from build123d import *

# Parameters (mm, degrees)
SKETCH1_R           = 4
BOSS_EXTRUDE1_DEPTH = 203.2
SKETCH2_R           = 1.864950538
CUT_EXTRUDE1_DEPTH  = 12.7
CUT_EXTRUDE2_START  = -6.35
CUT_EXTRUDE2_DEPTH  = 130.81


with BuildPart() as part:
    # Sketch1 → Boss-Extrude1 (new body)
    with BuildSketch(Plane(origin=(0, 0, 0), x_dir=(1, 0, 0), z_dir=(0, 1, 0))):
        with Locations(Location((0, 0, 0), (0, 0, 270))):
            Circle(SKETCH1_R)
    extrude(amount=BOSS_EXTRUDE1_DEPTH)

    # Sketch2 → Cut-Extrude1 (cut)
    with BuildSketch(Plane.XZ):
        with Locations(Location((0, 0, 0), (0, 0, 270))):
            Circle(SKETCH2_R)
    extrude(amount=-CUT_EXTRUDE1_DEPTH, mode=Mode.SUBTRACT)

    # Sketch4 → Cut-Extrude2 (cut)
    with BuildSketch(Plane.XZ.offset(CUT_EXTRUDE2_START)):
        Polygon((-31.691808684, 3.184149537), (-2.420989824, 3.184149537), (2.420989824, 3.184149537), (31.691808684, 3.184149537), (31.691808684, 61.725787257), (-31.691808684, 61.725787257), align=None)
    extrude(amount=-CUT_EXTRUDE2_DEPTH, mode=Mode.SUBTRACT)


solid = part.part
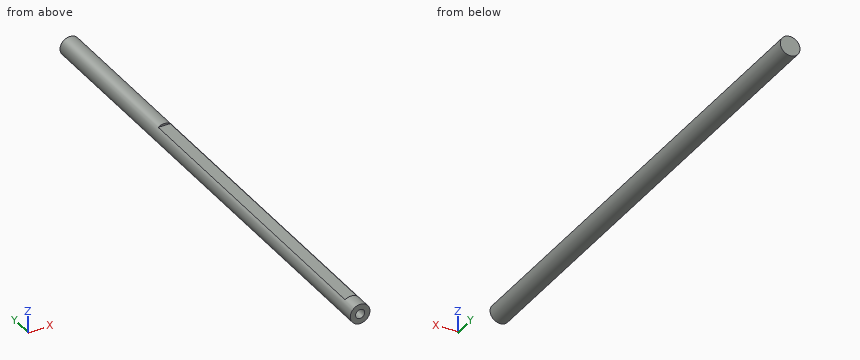
Geometry: final body of the model. Coordinates: model frame, mm. Coordinates: 2 decimals unless noted, no trailing zeros. Order: outer loops, then holes, each group sorted by start corner. A loop starts at its lowest first (then second) coordinate and runs counter-clockwise, first axis right, second up.
(1) Material intervals for probe 1 along X at (y, z) = (5.5, 0); probe 2 along Z at (x, y) = (0.25, 59); probe 3 along Y at (x, z) = (-1, -0.5), sorted ascending.
(2) Section query C-C (y = 183). Return the cut outline in (x, z).
(3) Section query A-A (z = 0). Return the cut outline in (x, y), plus the area to 3 significant figures.
(4) Section query B-B (x = 0). Return the cut outline in (y, z), plus the area to 3 significant figures.
(5) First-contact query: pin 1 (1.9 mm diameter, centred on x = 0, z = -0.5, fed in from -Y); pin 2 (2 mm diameter, centred on x = -3, y = 65, fed in from -Z); pin 3 (1.5 mm diameter, centred on x = -1, y = 60.5, fed in from +Z). Flat tips, straight axial feed; report the tip coordinate or a pass-through.
(6) Section query D-D (y = 83). Return the cut outline in (x, z).
Solution:
1. probe 1: x = -4 to -1.86, 1.86 to 4
1. probe 2: z = -3.99 to 3.18
1. probe 3: y = 12.7 to 203.2
2. outline: circle Ø8 at (0, 0)
3. outline: (-4, 0) - (-1.86, 0) - (-1.86, 12.7) - (1.86, 12.7) - (1.86, 0) - (4, 0) - (4, 203.2) - (-4, 203.2) - close
3. area: 1,580 mm2
4. outline: (0, -4) - (203.2, -4) - (203.2, 4) - (137.16, 4) - (137.16, 3.18) - (6.35, 3.18) - (6.35, 4) - (0, 4) - (0, 1.86) - (12.7, 1.86) - (12.7, -1.86) - (0, -1.86) - close
4. area: 1,470 mm2
5. pin 1: stops at y = 12.7
5. pin 2: stops at z = -3.46
5. pin 3: stops at z = 3.18
6. outline: (-2.42, 3.18) arc R4 ccw (long way) to (2.42, 3.18) - close
